The model under review builds one solid part; all positions refer to its coordinate system, in mm. Coordinates: 2 decimals unless noted, no trailing zeros. Loops run counter-clockwise (first coordinate to the right, second up) from the corner with the lowest first, then second, coordinate; pieces in that order, holes last. Notation, with made-up numbers: M -1.75,87.25 L 16.25,87.25 A8 cw 16.25,92.25 Z; hole C 68.25,20 d1. An arc over 180 degrees is marked long. Write item = value, one per line. Start each with the question number.
Q1. Wall thickness on probe 1 along X at (y, z) = (18, 0); probe 2 along Z at (x, y) = (-2.5, 23.5); probe 3 along Z at (x, y) = (-0.5, 2): over which ranges is each line inside the solid? List them lowest first.
Q2. Mouldability with a two-part tool opening along X and no side actions: class faces 1 (the face through (1.379, 22.192, -3.325)), 2 (the face through (2, 45, -4)), 3 (the face through (9.76, 22.19, 2.17)) as released by +X, released by -X, zero draft, split by the parting line, or undercut.
Q3. We need section C-C on y = 38.5. Give the boundary of the cut face in (x, z), and give its area (3 significant figures).
Q4. Clearance check with flat-ended pins moving along their axes: pin 1 Ø1.5 at (y, z) = (8, 4.5) entering from -X; pin 2 Ø8 at (y, z) = (21, 8) entering from -X; pin 3 Ø1 at (x, y) = (7, 11.5) entering from +Z. State where each tip first meets the part, or that it passes through.
Q5. We need section B-B on x = 0. Give the boundary of the cut face in (y, z), and give its area (3 significant figures).
Q6. We need section A-A on z = 0. Give the boundary of the cut face in (x, y), and give its area (3 significant figures).
from build123d import *

# Parameters (mm, degrees)
SKICA2_R                = 10
SKICA2_R_2              = 3.6
P_IDAT_VYSUNUT_M1_DEPTH = 45
ZKOSEN_1_SIZE           = 0.5


with BuildPart() as part:
    # Skica2 → Přidat vysunutím1 (new body)
    with BuildSketch(Plane(origin=(0, 0, 0), x_dir=(1, 0, 0), z_dir=(0, 1, 0))):
        with Locations(Location((0, 0, 0), (0, 0, 90))):
            Circle(SKICA2_R)
        with Locations(Location((0, 0, 0), (0, 0, 90))):
            Circle(SKICA2_R_2, mode=Mode.SUBTRACT)
    extrude(amount=P_IDAT_VYSUNUT_M1_DEPTH)

    # Zkosení1
    zkosen_1_edges = [part.edges().sort_by_distance(p)[0] for p in [
        (0, 0, 10),
        (0, 45, 10),
        (0, 0, 3.6),
        (0, 45, 3.6),
    ]]
    chamfer(zkosen_1_edges, length=ZKOSEN_1_SIZE)


solid = part.part
Returned:
q1.probe_1 = -10 to -3.6, 3.6 to 10
q1.probe_2 = -9.68 to -2.59, 2.59 to 9.68
q1.probe_3 = -9.99 to -3.57, 3.57 to 9.99
q2.face_1 = undercut
q2.face_2 = zero draft
q2.face_3 = split by the parting line
q3.outline = C 0,0 d20; hole C 0,0 d7.2
q3.area = 273 mm^2
q4.pin_1 = -9.27
q4.pin_2 = -9.17
q4.pin_3 = 7.6
q5.outline = M 0,-9.5 L 0.5,-10 L 44.5,-10 L 45,-9.5 L 45,-4.1 L 44.5,-3.6 L 0.5,-3.6 L 0,-4.1 Z; M 0,4.1 L 0.5,3.6 L 44.5,3.6 L 45,4.1 L 45,9.5 L 44.5,10 L 0.5,10 L 0,9.5 Z
q5.area = 575 mm^2
q6.outline = M -10,0.5 L -9.5,0 L -4.1,0 L -3.6,0.5 L -3.6,44.5 L -4.1,45 L -9.5,45 L -10,44.5 Z; M 3.6,0.5 L 4.1,0 L 9.5,0 L 10,0.5 L 10,44.5 L 9.5,45 L 4.1,45 L 3.6,44.5 Z
q6.area = 575 mm^2
